Source: CAD feature listing. Evaluate the final solid. Frame: model axes, mm. Give positions to 0.01 mm unless a question says otherwise; leave off trailing zeros. Use one line per item in the form item = value. Start each with the question number.
(1) Material intervals for line 1 along Z through (x, y) = (121.75, 1.95); line 2 along X through (y, z) = (1.9, 9); line 3 along X through (y, z) = (2.4, -15.25), sorted ascending. Write a range as from..to.
(2) Cut plane A-A, the plane y = 2.6. Count the separate pieces of the cut face and the enclosed holes in it, and give its area (3 significant figures).
(3) Draft query along X for faces 1 (the face through (69, 0, 0)), 2 (the face through (109, 2, -24.1)). Return one class per face: pulls with the +X half, pulls with the -X half, needs draft (parallel to the pull), parting line crosses it, or undercut.
(4) First-contact query: P1, Ø1.6, axis at x = 88.25, z = -9, coming from the +Y side. Flat tip, straight axial feed; report the tip coordinate or a pass-through.
from build123d import *

# Parameters (mm, degrees)
SKETCH1_W           = 140
SKETCH1_H           = 61
BOSS_EXTRUDE1_DEPTH = 4
SKETCH2_W           = 6
SKETCH2_H           = 20
CUT_EXTRUDE1_DEPTH  = 10
SKETCH4_3_R         = 1
SKETCH4_3_R_2       = 1.5
CUT_EXTRUDE3_DEPTH  = 4
CUT_EXTRUDE4_DEPTH  = 34
CUT_EXTRUDE5_DEPTH  = 10


with BuildPart() as part:
    # Sketch1 → Boss-Extrude1 (new body)
    with BuildSketch(Plane(origin=(0, 0, 0), x_dir=(1, 0, 0), z_dir=(0, 1, 0))):
        with Locations((70, 0)):
            Rectangle(SKETCH1_W, SKETCH1_H)
    extrude(amount=BOSS_EXTRUDE1_DEPTH)

    # Sketch2 → Cut-Extrude1 (cut)
    with BuildSketch(Plane(origin=(0, 4, 0), x_dir=(1, 0, 0), z_dir=(0, 1, 0))):
        with Locations((20.449723582, 11.650059082)):
            Rectangle(SKETCH2_W, SKETCH2_H)
    extrude(amount=-CUT_EXTRUDE1_DEPTH, mode=Mode.SUBTRACT)

    # Sketch4_3 → Cut-Extrude3 (cut)
    with BuildSketch(Plane.XZ):
        with Locations(Location((88.25, -9, 0), (0, 0, 270))):
            Circle(SKETCH4_3_R)
        with Locations(Location((88.25, 9, 0), (0, 0, 270))):
            Circle(SKETCH4_3_R)
        with Locations(Location((121.75, -9, 0), (0, 0, 270))):
            Circle(SKETCH4_3_R)
        with Locations(Location((121.75, 9, 0), (0, 0, 270))):
            Circle(SKETCH4_3_R)
        with Locations(Location((36.75, 15.25, 0), (0, 0, 270))):
            Circle(SKETCH4_3_R_2)
        with Locations(Location((67.25, 15.25, 0), (0, 0, 270))):
            Circle(SKETCH4_3_R_2)
        with Locations(Location((67.25, -15.25, 0), (0, 0, 270))):
            Circle(SKETCH4_3_R_2)
        with Locations(Location((36.75, -15.25, 0), (0, 0, 270))):
            Circle(SKETCH4_3_R_2)
    extrude(amount=-CUT_EXTRUDE3_DEPTH, mode=Mode.SUBTRACT)

    # Sketch6 → Cut-Extrude4 (cut)
    with BuildSketch(Plane(origin=(0, 4, 0), x_dir=(1, 0, 0), z_dir=(0, 1, 0))):
        Polygon((81.358539738, 14.6), (78.356318338, 14.6), (76.855207639, 12), (78.356318338, 9.4), (81.358539738, 9.4), (82.859650438, 12), align=None)
        Polygon((110.558539738, 5.1), (107.556318338, 5.1), (106.055207639, 2.5), (107.556318338, -0.1), (110.558539738, -0.1), (112.059650438, 2.5), align=None)
        Polygon((112.059650438, 21.5), (110.558539738, 24.1), (107.556318338, 24.1), (106.055207639, 21.5), (107.556318338, 18.9), (110.558539738, 18.9), align=None)
    extrude(amount=-CUT_EXTRUDE4_DEPTH, mode=Mode.SUBTRACT)

    # Sketch7 → Cut-Extrude5 (cut)
    with BuildSketch(Plane(origin=(0, 4, 0), x_dir=(1, 0, 0), z_dir=(0, 1, 0))):
        Polygon((9.961432148, -12.993206821), (8.90784571, -10.181927939), (5.946413563, -9.688721118), (4.038567852, -12.006793179), (5.09215429, -14.818072061), (8.053586437, -15.311278882), align=None)
        Polygon((135.961432148, -12.993206821), (134.90784571, -10.181927939), (131.946413563, -9.688721118), (130.038567852, -12.006793179), (131.09215429, -14.818072061), (134.053586437, -15.311278882), align=None)
    extrude(amount=-CUT_EXTRUDE5_DEPTH, mode=Mode.SUBTRACT)


solid = part.part
Geometry says:
q1.line_1 = -30.5..-10, -8..8, 10..30.5
q1.line_2 = 0..87.25, 89.25..120.75, 122.75..140
q1.line_3 = 0..17.45, 23.45..35.25, 38.25..65.75, 68.75..140
q2.separate_pieces = 1
q2.enclosed_holes = 14
q2.area = 8,260 mm^2
q3.face_1 = needs draft
q3.face_2 = undercut
q4.P1 = through
